Geometry check sheet. Reference: the model listing, model coordinates, mm. A direction names the side the tool comes from. Round coordinates to 2 decimals unless told otherwise and drop trailing zeros. Order: outer loops, then holes, each group sorted by start corner. A loop starts at its lowest first (then second) coordinate and runs counter-clockwise, first axis right, second up. Notation, with made-up numbers: (3.25, -9) - (59.25, -9) arc R21 cw to (59.25, 19) - close; hole circle Ø9 at (12.5, 89.25). An arc over 180 degrees is marked (long way). Use a Markdown table: item, result. Add a question column.
(1) Gauge pin test, flat end, axial feed: P1, Ø0.5, axis at y = -5.5, z = 3, coming from the +X side. Record the tip position at first contact, or that the pin passes through.
(2) Section check A-A on x = 0. Record the boundary of the cut face in (y, z).
(3) Section check C-C on z = 2.6. Record the boundary of the cut face in (x, y) (1 decimal).
(4) Section check D-D on z = 1.75. Record the boundary of the cut face in (x, y).
(5) Access from +Z, -Z, +X, -X, +Y, -Y to the whole of each face (thin tool, end or side, straight path). Record for faces 1 (the face through (-1.588, -7, 3)), 2 (the face through (0.035, 1.587, 3.273)), 3 (the face through (1.588, -8, 3)).
(6) Section check B-B on y = -4.75. Record the boundary of the cut face in (x, z).
(7) Thickness scan on line 1 along Z through (x, y) = (-1.9, -15); line 2 along X through (y, z) = (-4.5, 3.95); line 3 along Y through (x, z) = (-0.45, 1.55). Record the ranges inside material, lowest first. Write a range as [from, to].
```python
from build123d import *

# Parameters (mm, degrees)
BOSS_EXTRUDE1_DEPTH = 2.38125
BOSS_EXTRUDE2_DEPTH = 4.191


with BuildPart() as part:
    # Sketch1 → Boss-Extrude1 (new body)
    with BuildSketch(Plane.XY):
        with BuildLine():
            Line((2.38125, -14.859), (2.38125, 0))
            ThreePointArc((2.38125, 0), (0, 2.38125), (-2.38125, 0))
            Line((-2.38125, 0), (-2.38125, -14.859))
            ThreePointArc((-2.38125, -14.859), (0, -17.24025), (2.38125, -14.859))
        make_face()
        with BuildLine():
            Line((1.5875, -14.859), (1.5875, 0))
            ThreePointArc((1.5875, 0), (0, 1.5875), (-1.5875, 0))
            Line((-1.5875, 0), (-1.5875, -14.859))
            ThreePointArc((-1.5875, -14.859), (0, -16.4465), (1.5875, -14.859))
        make_face(mode=Mode.SUBTRACT)
    extrude(amount=BOSS_EXTRUDE1_DEPTH)

    # Sketch1<5> → Boss-Extrude2 (add)
    with BuildSketch(Plane.XY):
        with BuildLine():
            Line((1.5875, -14.859), (1.5875, 0))
            ThreePointArc((1.5875, 0), (0, 1.5875), (-1.5875, 0))
            Line((-1.5875, 0), (-1.5875, -14.859))
            ThreePointArc((-1.5875, -14.859), (0, -16.4465), (1.5875, -14.859))
        make_face()
    extrude(amount=BOSS_EXTRUDE2_DEPTH)


solid = part.part
```
Check sheet entries:
| question | item | result |
|---|---|---|
| 1 | P1 | stops at x = 1.59 |
| 2 | outline | (-17.24, 0) - (2.38, 0) - (2.38, 2.38) - (1.59, 2.38) - (1.59, 4.19) - (-16.45, 4.19) - (-16.45, 2.38) - (-17.24, 2.38) - close |
| 3 | outline | (-1.6, -14.9) arc R1.6 ccw to (1.6, -14.9) - (1.6, 0) arc R1.6 ccw to (-1.6, 0) - close |
| 4 | outline | (-2.38, -14.86) arc R2.38 ccw to (2.38, -14.86) - (2.38, 0) arc R2.38 ccw to (-2.38, 0) - close |
| 5 | face 1 | +Z, -X, +Y, -Y |
| 5 | face 2 | +Z, +Y |
| 5 | face 3 | +Z, +X, +Y, -Y |
| 6 | outline | (-2.38, 0) - (2.38, 0) - (2.38, 2.38) - (1.59, 2.38) - (1.59, 4.19) - (-1.59, 4.19) - (-1.59, 2.38) - (-2.38, 2.38) - close |
| 7 | line 1 | z = [0, 2.38] |
| 7 | line 2 | x = [-1.59, 1.59] |
| 7 | line 3 | y = [-17.2, 2.34] |
